Input: part model. Units: mm. Frame: model coordinates. A direction names the side the tool comes from. Round coordinates to 2 decimals unless told otherwise and drop trailing zeros. Order: outer loops, then holes, each group sorted by start corner. A loop starts at its lowest first (then second) coordinate and runs counter-clockwise, first axis right, second up. Notation, with made-up numbers: M 56,89.25 L 61,89.25 A25 ccw 61,114.25 Z; hole C -12,56 d3. An arc over 180 degrees is marked long. One line per question, with ' | ' between items.
```python
from build123d import *

# Parameters (mm, degrees)
SKETCH1_W           = 25
SKETCH1_H           = 27
SKETCH1_W_2         = 21
SKETCH1_H_2         = 23
BOSS_EXTRUDE1_DEPTH = 11
CUT_EXTRUDE1_START  = -10.5
SKETCH2_W           = 10
SKETCH2_H           = 17
CUT_EXTRUDE1_DEPTH  = 3


with BuildPart() as part:
    # Sketch1 → Boss-Extrude1 (new body, symmetric)
    with BuildSketch(Plane(origin=(0, 0, 0), x_dir=(1, 0, 0), z_dir=(0, 1, 0))):
        Rectangle(SKETCH1_W, SKETCH1_H)
        Rectangle(SKETCH1_W_2, SKETCH1_H_2, mode=Mode.SUBTRACT)
    extrude(amount=BOSS_EXTRUDE1_DEPTH, both=True)

    # Sketch2 → Cut-Extrude1 (cut)
    with BuildSketch(Plane(origin=(0, 0, 0), x_dir=(0, 0, -1), z_dir=(1, 0, 0)).offset(CUT_EXTRUDE1_START)):
        with Locations((0, 2.5)):
            Rectangle(SKETCH2_W, SKETCH2_H)
    extrude(amount=-CUT_EXTRUDE1_DEPTH, mode=Mode.SUBTRACT)


solid = part.part
```
Item 1: Access query for faces 5 (the flat face through (-11, -11, 0)), 6 (the flat face through (0, 0, -11.5)), 7 (the flat face through (-11, 2, 5)). Directions: +Z, -Z, +X, -X, +Y, -Y. A direction counts if a zero-diameter tool reaches every point of the face in a straight line with its end or side. Return the directions, or none.
Report:
face 5: +Z, -Z, +X, -X, -Y | face 6: +Y, -Y | face 7: -X, +Y
Item 2: Section query B-B, the plane y = -9.25. Return loops of the section in (x, z), plus the area to 3 significant figures.
Report:
outline: M -12.5,-13.5 L 12.5,-13.5 L 12.5,13.5 L -12.5,13.5 Z; hole M -10.5,-11.5 L 10.5,-11.5 L 10.5,11.5 L -10.5,11.5 Z | area: 192 mm²
Item 3: Section query D-D, the plane y = -3. Return loops of the section in (x, z), plus the area to 3 significant figures.
Report:
outline: M -12.5,-13.5 L 12.5,-13.5 L 12.5,13.5 L -12.5,13.5 L -12.5,5 L -10.5,5 L -10.5,11.5 L 10.5,11.5 L 10.5,-11.5 L -10.5,-11.5 L -10.5,-5 L -12.5,-5 Z | area: 172 mm²
Item 4: Section query A-A, the plane x = -8. Return loops of the section in (y, z), plus the area to 3 significant figures.
Report:
outline: M -11,-13.5 L 11,-13.5 L 11,-11.5 L -11,-11.5 Z; M -11,11.5 L 11,11.5 L 11,13.5 L -11,13.5 Z | area: 88.0 mm²
Item 5: Section query C-C, the plane z = 4. Return loops of the section in (x, y), plus the area to 3 significant figures.
Report:
outline: M -12.5,-11 L -10.5,-11 L -10.5,-6 L -12.5,-6 Z; M 10.5,-11 L 12.5,-11 L 12.5,11 L 10.5,11 Z | area: 54.0 mm²
Item 6: First-contact query: pin 1 (12 mm diameter, centred on x = 1.5, z = -4, fed in from -Y); pin 2 (1 mm diameter, centred on x = -11, z = 1.5, fed in from +Y). Flat tips, straight axial feed; report the tip coordinate or a pass-through.
Report:
pin 1: through | pin 2: y = -6
Item 7: Line query: line 1 along Z through (x, y) = (9.75, -1.5); line 2 along X through (y, z) = (-6.5, 4.25); line 3 along X through (y, z) = (2.25, -3.5). Output: solid intervals per line, ascending. Write a range as from..to.
Report:
line 1: -13.5..-11.5, 11.5..13.5 | line 2: -12.5..-10.5, 10.5..12.5 | line 3: 10.5..12.5
Item 8: Mould query, pull axis X, two halves, no side actions, for faces 1 (the flat face through (-10.5, -2.3, 5.3)), 2 (the flat face through (10.5, 0, 0)), 3 (the flat face through (11, 11, 1)), 4 (the flat face through (-12.5, 0, -6)). Classes: +X half, -X half, draft (parallel to the pull), parting line (faces both ways), or undercut.
Report:
face 1: undercut | face 2: undercut | face 3: draft | face 4: -X half
